Geometry check sheet. Reference: the model listing, model coordinates, mm. Face numbers are marked on the shaded views. A direction names the side the tool comes from. Round coordinates to 2 decimals unless told otherwise and drop trailing zeros. Order: outer loops, then holes, each group sorted by start corner. A loop starts at its lowest first (then second) coordinate and runs counter-clockwise, first axis right, second up. Notation, with made-up numbers: (-18, -23) - (-1, -23) arc R18 ccw to (-1, -2) - close; hole circle Ø1 at (10.25, -31.5). An arc over 180 degrees is marked (long way). One line per question, with ' | ' between items. Start each with the question number.
Q1. Gauge pin test, flat ends, axial feed: P1, Ø3.5, axis at y = 9.5, z = 31, coming from the +X side; P2, Ø6.5, axis at y = 10, z = 30, coming from the -X side. Record the tip position at first contact, or that the pin passes through.
Q2. Sectioned sample at B-B, the plane z = 30. Enter the section's corners in (x, y).
Q3. Mould release check, pull along Z, two halves, no side actions. Record for the marked faces 1, 2 and 3: +Z half, -Z half, draft (parallel to the pull), parting line (faces both ways), or undercut.
Q4. Sectioned sample at C-C, the plane x = 8.75. Enter the section's corners in (y, z).
Q5. Sectioned sample at D-D, the plane x = 4.5. Enter the section's corners in (y, z), then the cut area to 3 significant figures.
Q6. Sectioned sample at A-A, the plane y = -10. Enter the section's corners in (x, z), then the cut area to 3 significant figures.
Q7. Tool access check on the marked faces 4 and 5. Record the directions out of +Z, -Z, +X, -X, +Y, -Y that give a thin tool (end or side, any length) a straight path to the whole face; none if there is none.
Q8. Material ranges on line 1 along Y through (x, z) = (8, 5); line 2 along Y through (x, z) = (3.95, 5); line 3 along Z through (x, y) = (8, -12.5), recorded low to high.
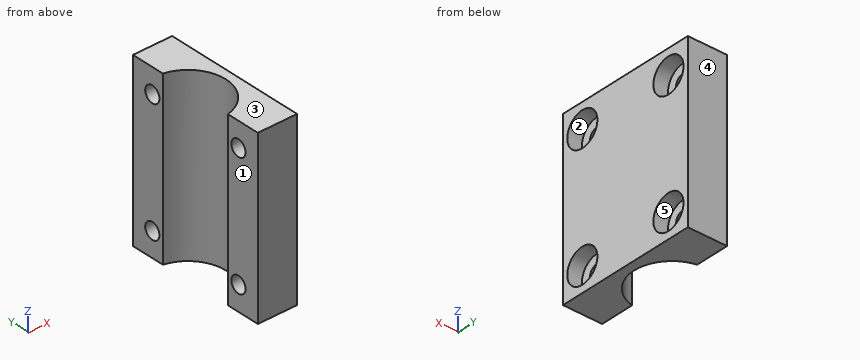
```python
from build123d import *

# Parameters (mm, degrees)
ESBO_O2_R                  = 7.7
ESBO_O2_W                  = 7
ESBO_O2_H                  = 10
RESSALTO_EXTRUS_O1_DEPTH   = 35
ESBO_O3_R                  = 1.65
CORTE_EXTRUS_O1_DEPTH      = 20
ESBO_O4_R                  = 1.6
CORTE_EXTRUS_O2_DEPTH      = 18.5
CORTE_EXTRUS_O2_DEPTH_BACK = 48.5
CORTE_EXTRUS_O4_START      = -8
ESBO_O8_W                  = 35
ESBO_O8_H                  = 65
CORTE_EXTRUS_O4_DEPTH      = 39
ESBO_O11_W                 = 8
ESBO_O11_H                 = 18
CORTE_EXTRUS_O6_DEPTH      = 1
CORTE_EXTRUS_O6_DEPTH_BACK = 36
ESBO_O12_R                 = 3.5
CORTE_EXTRUS_O7_DEPTH      = 3


with BuildPart() as part:
    # Esboço2 → Ressalto-extrusão1 (new body)
    with BuildSketch(Plane.XY):
        Polygon((-9.5, 15), (-9.5, 32.5), (9.5, 32.5), (9.5, -32.5), (-9.5, -32.5), (-9.5, -15), (-25, -15), (-25, -12), (-9, -12), (-9, -2), (-25, -2), (-36.5, -2), (-36.5, 2), (-20.5, 2), (-20.5, 12), (-36.5, 12), (-36.5, 15), align=None)
        Circle(ESBO_O2_R, mode=Mode.SUBTRACT)
        with Locations((-12.5, 7)):
            Rectangle(ESBO_O2_W, ESBO_O2_H, mode=Mode.SUBTRACT)
    extrude(amount=RESSALTO_EXTRUS_O1_DEPTH)

    # Esboço3 → Corte-extrusão1 (cut, through all)
    with BuildSketch(Plane.ZY.offset(9.5)):
        with Locations((17.5, 18)):
            Circle(ESBO_O3_R)
        with Locations((17.5, -18)):
            Circle(ESBO_O3_R)
        with Locations((5, 10)):
            Circle(ESBO_O3_R)
        with Locations((30, 10)):
            Circle(ESBO_O3_R)
        with Locations((5, -10)):
            Circle(ESBO_O3_R)
        with Locations((30, -10)):
            Circle(ESBO_O3_R)
        Polygon((35, 30.736730193), (25, 32.5), (35, 32.5), align=None)
        Polygon((24.739796996, 20.169435313), (30.057758862, 19.231735154), (29.536814329, 16.277311895), (24.218852463, 17.215012054), align=None)
        with BuildLine():
            Line((21.321510517, 23.818451283), (42.639721186, 20.059475562))
            Line((42.639721186, 20.059475562), (42.813369364, 21.044283315))
            Line((42.813369364, 21.044283315), (21.495158694, 24.803259036))
            ThreePointArc((21.495158694, 24.803259036), (13.560768988, 25.694592711), (21.321510517, 23.818451283))
        make_face()
        with BuildLine():
            Line((42.639721186, -20.059475562), (42.813369364, -21.044283315))
            Line((42.813369364, -21.044283315), (21.495158694, -24.803259036))
            ThreePointArc((21.495158694, -24.803259036), (13.560768988, -25.694592711), (21.321510517, -23.818451283))
            Line((21.321510517, -23.818451283), (42.639721186, -20.059475562))
        make_face()
        Polygon((30.057758862, -19.231735154), (29.536814329, -16.277311895), (24.218852463, -17.215012054), (24.739796996, -20.169435313), align=None)
        Polygon((0, 30.736730193), (10, 32.5), (0, 32.5), align=None)
        Polygon((35, -32.5), (25, -32.5), (35, -30.736730193), align=None)
        Polygon((0, -32.5), (10, -32.5), (0, -30.736730193), align=None)
    extrude(amount=-CORTE_EXTRUS_O1_DEPTH, mode=Mode.SUBTRACT)

    # Esboço4 → Corte-extrusão2 (cut, two sides)
    with BuildSketch(Plane(origin=(0, 15, 0), x_dir=(1, 0, 0), z_dir=(0, 1, 0))) as corte_extrus_o2_sk:
        with Locations((-32, -11.5)):
            Circle(ESBO_O4_R)
        with Locations((-19, -23.5)):
            Circle(ESBO_O4_R)
    extrude(amount=CORTE_EXTRUS_O2_DEPTH, mode=Mode.SUBTRACT)
    extrude(corte_extrus_o2_sk.sketch, amount=-CORTE_EXTRUS_O2_DEPTH_BACK, mode=Mode.SUBTRACT)

    # Esboço8 → Corte-extrusão4 (cut, through all)
    with BuildSketch(Plane(origin=(9.5, 0, 0), x_dir=(0, 0, -1), z_dir=(1, 0, 0)).offset(CORTE_EXTRUS_O4_START)):
        with Locations((-17.5, 0)):
            Rectangle(ESBO_O8_W, ESBO_O8_H)
    extrude(amount=-CORTE_EXTRUS_O4_DEPTH, mode=Mode.SUBTRACT)

    # Esboço11 → Corte-extrusão6 (cut, two sides)
    with BuildSketch(Plane(origin=(0, 0, 0), x_dir=(-1, 0, 0), z_dir=(0, 0, -1))) as corte_extrus_o6_sk:
        with Locations((-5.5, 23.5)):
            Rectangle(ESBO_O11_W, ESBO_O11_H)
        with Locations((-5.5, -23.5)):
            Rectangle(ESBO_O11_W, ESBO_O11_H)
    extrude(amount=CORTE_EXTRUS_O6_DEPTH, mode=Mode.SUBTRACT)
    extrude(corte_extrus_o6_sk.sketch, amount=-CORTE_EXTRUS_O6_DEPTH_BACK, mode=Mode.SUBTRACT)

    # Esboço12 → Corte-extrusão7 (cut)
    with BuildSketch(Plane(origin=(9.5, 0, 0), x_dir=(0, 0, -1), z_dir=(1, 0, 0))):
        with Locations((-30, 10)):
            Circle(ESBO_O12_R)
        with Locations((-5, 10)):
            Circle(ESBO_O12_R)
        with Locations((-5, -10)):
            Circle(ESBO_O12_R)
        with Locations((-30, -10)):
            Circle(ESBO_O12_R)
    extrude(amount=-CORTE_EXTRUS_O7_DEPTH, mode=Mode.SUBTRACT)


solid = part.part
```
Determined:
1) P1: stops at x = 6.5 | P2: stops at x = 1.5
2) outline: (1.5, -14.5) - (9.5, -14.5) - (9.5, -13.5) - (6.5, -13.5) - (6.5, -11.65) - (1.5, -11.65) - close; (1.5, -8.35) - (6.5, -8.35) - (6.5, -6.5) - (9.5, -6.5) - (9.5, 6.5) - (6.5, 6.5) - (6.5, 8.35) - (1.5, 8.35) - (1.5, 7.55) arc R7.7 cw to (1.5, -7.55) - close; (1.5, 11.65) - (6.5, 11.65) - (6.5, 13.5) - (9.5, 13.5) - (9.5, 14.5) - (1.5, 14.5) - close
3) face 1: draft | face 2: undercut | face 3: +Z half
4) outline: (-14.5, 0) - (14.5, 0) - (14.5, 35) - (-14.5, 35) - close; hole circle Ø7 at (-10, 5); hole circle Ø7 at (-10, 30); hole circle Ø7 at (10, 5); hole circle Ø7 at (10, 30)
5) outline: (-14.5, 0) - (-6.25, 0) - (-6.25, 35) - (-14.5, 35) - close; (6.25, 0) - (14.5, 0) - (14.5, 35) - (6.25, 35) - close; hole circle Ø3.3 at (-10, 5); hole circle Ø3.3 at (-10, 30); hole circle Ø3.3 at (10, 5); hole circle Ø3.3 at (10, 30) | area: 543 mm2
6) outline: (1.5, 0) - (9.5, 0) - (9.5, 1.5) - (6.5, 1.5) - (6.5, 3.35) - (1.5, 3.35) - close; (1.5, 6.65) - (6.5, 6.65) - (6.5, 8.5) - (9.5, 8.5) - (9.5, 26.5) - (6.5, 26.5) - (6.5, 28.35) - (1.5, 28.35) - close; (1.5, 31.65) - (6.5, 31.65) - (6.5, 33.5) - (9.5, 33.5) - (9.5, 35) - (1.5, 35) - close | area: 205 mm2
7) face 4: +Z, -Z, +X, -X, +Y | face 5: +X
8) line 1: y = -14.5 to -13.5, -6.5 to 6.5, 13.5 to 14.5 | line 2: y = -14.5 to -11.65, -8.35 to -6.61, 6.61 to 8.35, 11.65 to 14.5 | line 3: z = 0 to 2.55, 7.45 to 27.55, 32.45 to 35
